Could you check a few things on this model? Use its own coordinates, in mm. A direction names the side the tool comes from. Coordinates: 2 decimals unless noted, no trailing zeros. Loops run counter-clockwise (first coordinate to the right, second up) from the corner with the lowest first, then second, coordinate; pieces in that order, holes last.
from build123d import *

# Parameters (mm, degrees)
SKETCH1_R                   = 3
BOSS_EXTRUDE1_DEPTH         = 32
TAP_DRILL_FOR_M3_TAP1_D     = 2.5
TAP_DRILL_FOR_M3_TAP1_DEPTH = 10
TAP_DRILL_FOR_M3_TAP1_TIP   = 0.751075774
TAP_DRILL_FOR_M3_TAP2_D     = 2.5
TAP_DRILL_FOR_M3_TAP2_DEPTH = 10
TAP_DRILL_FOR_M3_TAP2_TIP   = 0.751075774


with BuildPart() as part:
    # Sketch1 → Boss-Extrude1 (new body)
    with BuildSketch(Plane(origin=(0, 0, 0), x_dir=(1, 0, 0), z_dir=(0, 1, 0))):
        Circle(SKETCH1_R)
    extrude(amount=BOSS_EXTRUDE1_DEPTH)

    # Tap Drill for M3 Tap1
    with Locations(Plane(origin=(0, 32, 0), x_dir=(1, 0, 0), z_dir=(0, 1, 0))):
        with Locations((0, 0)):
            Hole(TAP_DRILL_FOR_M3_TAP1_D / 2, depth=TAP_DRILL_FOR_M3_TAP1_DEPTH)
            with Locations((0, 0, -(TAP_DRILL_FOR_M3_TAP1_DEPTH + TAP_DRILL_FOR_M3_TAP1_TIP / 2))):  # 118° drill point
                Cone(0, TAP_DRILL_FOR_M3_TAP1_D / 2, TAP_DRILL_FOR_M3_TAP1_TIP, mode=Mode.SUBTRACT)

    # Tap Drill for M3 Tap2
    with Locations(Plane(origin=(0, 0, 0), x_dir=(-1, 0, 0), z_dir=(0, -1, 0))):
        with Locations((0, 0)):
            Hole(TAP_DRILL_FOR_M3_TAP2_D / 2, depth=TAP_DRILL_FOR_M3_TAP2_DEPTH)
            with Locations((0, 0, -(TAP_DRILL_FOR_M3_TAP2_DEPTH + TAP_DRILL_FOR_M3_TAP2_TIP / 2))):  # 118° drill point
                Cone(0, TAP_DRILL_FOR_M3_TAP2_D / 2, TAP_DRILL_FOR_M3_TAP2_TIP, mode=Mode.SUBTRACT)


solid = part.part
(1) Imagine slicing it at A-A, the plane y = 22.5. Write out the boundary of the cut face in (x, z).
Answers:
outline: circle Ø6 at (0, 0); hole circle Ø2.5 at (0, 0)
(2) We'd pull the mould along Z, two halves only. Please class faces 1 (the face through (-3, 16, 0)), 2 (the face through (0.05, 10.62, 0.21)), 3 (the face through (1, 32, 1)): +Z half, -Z half, draft (parallel to the pull), parting line (faces both ways), or undercut.
Answers:
face 1: parting line
face 2: undercut
face 3: draft
(3) Which directions (+Z, -Z, +X, -X, +Y, -Y) give clear straight access to the entire face, cutting with the end or side of a thin tool? Please do faces 4 (the face through (1, 0, 1)), 5 (the face through (-0.27, 5.07, 1.22)), 6 (the face through (0.27, 26.93, 1.22)).
Answers:
face 4: +Z, -Z, +X, -X, -Y
face 5: -Y
face 6: +Y
(4) I need wall thicknesses on probe 1 along Z at (x, y) = (0, 26.25); probe 2 along X at (y, z) = (17, 0.15); probe 3 along Z at (x, y) = (-0.7, 9). Which ranges of each line are inside material? Lowest first, please.
Answers:
probe 1: z = -3 to -1.25, 1.25 to 3
probe 2: x = -3 to 3
probe 3: z = -2.92 to -1.04, 1.04 to 2.92
(5) Imagine slicing it at B-B, the plane z = 2.4. Write out the boundary of the cut face in (x, y), and give its area (3 significant figures).
Answers:
outline: (-1.8, 0) - (1.8, 0) - (1.8, 32) - (-1.8, 32) - close
area: 115 mm2
(6) Imagine slicing it at C-C, the plane x = -1.95. Write out the boundary of the cut face in (y, z).
Answers:
outline: (0, -2.28) - (32, -2.28) - (32, 2.28) - (0, 2.28) - close
(7) For pin 1 (3 mm diameter, centred on x = 0, z = 0, fed in from +Y); pin 2 (1 mm diameter, centred on x = 1.5, y = 5.5, fed in from -Z); pin 3 (1.5 mm diameter, centred on x = 0, z = 0, fed in from -Y), each with a flat end and sliding along its axis, tell me the tip position at first contact or that it passes through.
Answers:
pin 1: stops at y = 32
pin 2: stops at z = -2.83
pin 3: stops at y = 10.3
